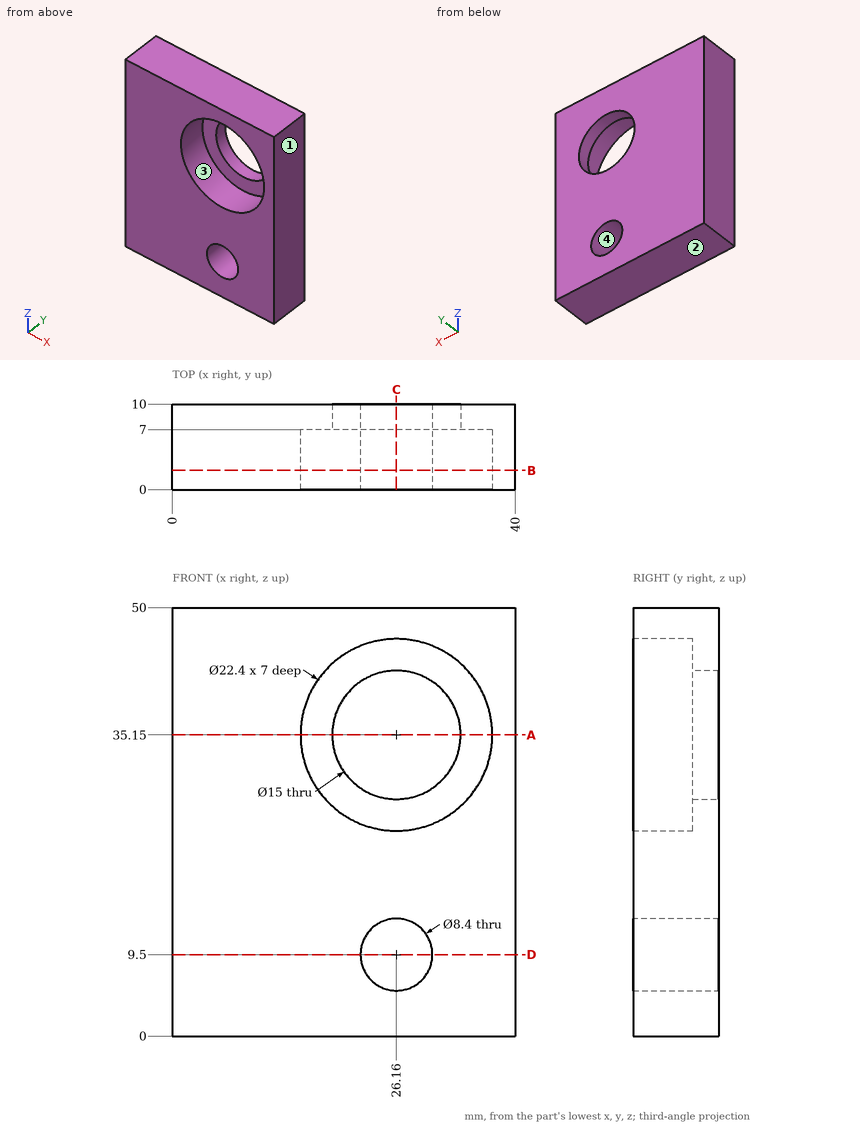
Answer from the drawing. Dimensions are ordinates in mm from the lowest x, y and z of the part. Round coordinates to 2 decimals unless told otherwise and drop trailing zeros. Write each loop counter-clockwise with the first axis right and the second up, starting at its lowest first coordinate (ties: lowest second). Pieces come first, ordered by that corner, then holes. Notation, with made-up numbers: (43.5, 50) -> (71.5, 50) arc R18 cw to (71.5, 78) -> close; hole circle Ø4 at (74.5, 28.5). An arc over 180 degrees is marked (long way). Answer in a Markdown table with one row per item. Add a question column.
1) Given P1, Ø1, axis at x = 29.5, z = 5, coming from the -Y side; P2, Ø12, axis at x = 26.16, z = 35.15, coming from the +Y side, each flat-ended and moving along its own axis, determine where each tip first touches the part or whether it passes through.
2) Determine the mould class of the marked faces 1, 2, 3 and 4 for opening direction X: pulls with the +X half, pulls with the -X half, needs draft (parallel to the pull), parting line crosses it, or undercut.
3) Find section D-D, the plane z = 9.5. Determine the outline of the cut face in (x, y).
4) Find section B-B, the plane y = 2.25. Determine the outline of the cut face in (x, z).
5) Find section A-A, the plane z = 35.15. Determine the outline of the cut face in (x, y), and give its area (3 significant figures).
6) Find section C-C, the plane x = 26.16. Determine the outline of the cut face in (y, z), and give its area (3 significant figures).
7) Consider line 1 (Z direction, x = 26, y = 6.5); line 2 (X direction, y = 2.5, z = 9.5); line 3 (X direction, y = 7.7, z = 35.15). Determine where each line is inside the solid, lowest interval first.
Findings below:
| question | item | result |
|---|---|---|
| 1 | P1 | y = 0 |
| 1 | P2 | through |
| 2 | face 1 | pulls with the +X half |
| 2 | face 2 | needs draft |
| 2 | face 3 | undercut |
| 2 | face 4 | undercut |
| 3 | outline | (0, 0) -> (21.96, 0) -> (21.96, 10) -> (0, 10) -> close; (30.36, 0) -> (40, 0) -> (40, 10) -> (30.36, 10) -> close |
| 4 | outline | (0, 0) -> (40, 0) -> (40, 50) -> (0, 50) -> close; hole circle Ø22.4 at (26.16, 35.15); hole circle Ø8.4 at (26.16, 9.5) |
| 5 | outline | (0, 0) -> (14.96, 0) -> (14.96, 7) -> (18.66, 7) -> (18.66, 10) -> (0, 10) -> close; (33.66, 7) -> (37.36, 7) -> (37.36, 0) -> (40, 0) -> (40, 10) -> (33.66, 10) -> close |
| 5 | area | 198 mm² |
| 6 | outline | (0, 0) -> (10, 0) -> (10, 5.3) -> (0, 5.3) -> close; (0, 13.7) -> (10, 13.7) -> (10, 27.65) -> (7, 27.65) -> (7, 23.95) -> (0, 23.95) -> close; (0, 46.35) -> (7, 46.35) -> (7, 42.65) -> (10, 42.65) -> (10, 50) -> (0, 50) -> close |
| 6 | area | 214 mm² |
| 7 | line 1 | 0 to 5.3, 13.7 to 23.95, 46.35 to 50 |
| 7 | line 2 | 0 to 21.96, 30.36 to 40 |
| 7 | line 3 | 0 to 18.66, 33.66 to 40 |
